Check sheet for the modelled part. Datum: model origin and axes. Units: mm. Face numbers are marked on the shaded views. A direction names the side the tool comes from. Round coordinates to 2 decimals unless told otherwise and drop trailing zeros. Write each loop counter-clockwise with the first axis right and the second up, starting at its lowest first coordinate (ties: lowest second). Pieces come first, ordered by that corner, then holes. Notation, with made-up numbers: (19.25, 15) - (36.25, 15) arc R21 ccw to (36.25, 45) - close; hole circle Ø7 at (-6, 85.5). An arc over 180 degrees is marked (long way). Use one line per item in the form item = value. Start each with the question number.
1) Section check B-B (x = 0). Record the boundary of the cut face in (y, z), then the cut area to 3 significant figures.
2) Set-up check for the marked faces 1 and 2: record each of +Z, -Z, +X, -X, +Y, -Y from which the full face is reachable in a straight line by a thin tool's end or side.
3) Section check C-C (x = -10). Record the boundary of the cut face in (y, z).
4) Section check D-D (y = 0.5). Record the boundary of the cut face in (x, z), then the cut area to 3 significant figures.
5) Draft check along X on the marked faces 3, 4 and 5. Enter one of: +X half, -X half, draft (parallel to the pull), parting line (faces both ways), or undercut.
6) Section check A-A (y = 5.5). Record the boundary of the cut face in (x, z).
7) Gauge pin test, flat ends, axial feed: P1, Ø3, axis at x = 8.5, y = 6.5, coming from the +Z side; P2, Ø3.5, axis at x = -1.5, y = 4.5, coming from the -Z side; P3, Ø1.5, axis at y = 2, z = 6, coming from the -X side. Record the tip position at first contact, or that the pin passes through.
8) Scan lines: probe 1 along X at (y, z) = (6, 0); probe 2 along Z at (x, y) = (0, 6.75); probe 3 along X at (y, z) = (1.25, 0.5). Record each from-to range of solid material in increasing order.
from build123d import *

# Parameters (mm, degrees)
CUT_EXTRUDE1_DEPTH = 24.28364121


with BuildPart() as part:
    # Sketch3 → Revolve1 (revolve)
    with BuildSketch(Plane(origin=(0, 0, 0), x_dir=(0, 0, -1), z_dir=(1, 0, 0))):
        Polygon((0, 7.874), (14.2748, 7.874), (14.2748, 1.651), (15.494, 1.651), (15.494, 0), (0, 0), align=None)
    revolve(axis=Axis((0, 0, 0), (0, 1, 0)))

    # Sketch4 → Cut-Extrude1 (cut, through all)
    with BuildSketch(Plane(origin=(0, 7.874, 0), x_dir=(1, 0, 0), z_dir=(0, 1, 0))):
        Polygon((-3.666174209, 6.35), (-7.332348419, 0), (-3.666174209, -6.35), (3.666174209, -6.35), (7.332348419, 0), (3.666174209, 6.35), align=None)
    extrude(amount=-CUT_EXTRUDE1_DEPTH, mode=Mode.SUBTRACT)


solid = part.part
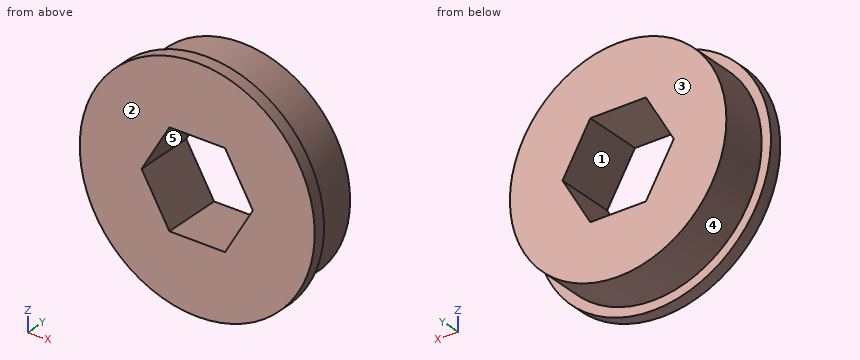
Results are:
q1.outline = (0, -15.49) - (1.65, -15.49) - (1.65, -14.27) - (7.87, -14.27) - (7.87, -6.35) - (0, -6.35) - close; (0, 6.35) - (7.87, 6.35) - (7.87, 14.27) - (1.65, 14.27) - (1.65, 15.49) - (0, 15.49) - close
q1.area = 129 mm²
q2.face_1 = +Y, -Y
q2.face_2 = +Z, -Z, +X, -X, -Y
q3.outline = (0, -11.83) - (1.65, -11.83) - (1.65, -10.19) - (7.87, -10.19) - (7.87, 10.19) - (1.65, 10.19) - (1.65, 11.83) - (0, 11.83) - close
q4.outline = circle Ø30.99 at (0, 0); hole (-7.33, 0) - (-3.67, -6.35) - (3.67, -6.35) - (7.33, 0) - (3.67, 6.35) - (-3.67, 6.35) - close
q4.area = 615 mm²
q5.face_3 = draft
q5.face_4 = parting line
q5.face_5 = undercut
q6.outline = circle Ø28.55 at (0, 0); hole (-7.33, 0) - (-3.67, -6.35) - (3.67, -6.35) - (7.33, 0) - (3.67, 6.35) - (-3.67, 6.35) - close
q7.P1 = 12.44
q7.P2 = -14.27
q7.P3 = -14.55
q8.probe_1 = -14.27 to -7.33, 7.33 to 14.27
q8.probe_2 = -14.27 to -6.35, 6.35 to 14.27
q8.probe_3 = -15.49 to -7.04, 7.04 to 15.49
